Geometry check sheet. Reference: the model listing, model coordinates, mm. A direction names the side the tool comes from. Give positions to 0.01 mm unless a question says otherwise; leave off trailing zeros. Loops run counter-clockwise (first coordinate to the right, second up) from the corner with the lowest first, then second, coordinate; pieces in that order, holes last. Notation, with made-up numbers: (50.5, 23) -> (97.5, 23) arc R18 ccw to (97.5, 35) -> close; hole circle Ø5 at (71, 19). An arc over 180 degrees is marked (long way). One line per item, written item: value. Start each with the question number.
(1) Gauge pin test, flat ends, axial feed: pin 1 Ø2 at (x, z) = (164.35, 11.66) entering from +Y; pin 2 Ø4 at (y, z) = (2, -79) entering from +X; pin 3 Ø10.5 at (x, z) = (183, 0.5) entering from +Y; pin 4 Ø7.5 at (x, z) = (182.175, 0) entering from +Y. Record the tip position at first contact, or that the pin passes through.
(2) Scan lines: line 1 along Z through (x, y) = (23, 2.75) (3 decimals); line 2 along X through (y, z) = (0.5, -80) (3 decimals); line 3 along X through (y, z) = (7.25, 9.5). Record each from-to range of solid material in increasing order. Write a range as from..to.
(3) Sectioned sample at B-B, the plane z = -33.5. Record the cut outline in (x, y), then the cut area to 3 significant figures.
(4) Sectioned sample at A-A, the plane x = 1. Record the cut outline in (y, z) (3 decimals).
(5) Draft check along Z on faces 1 (the face through (146.106, 3.944, 46.261)), 2 (the face through (85, 0, 1)), 3 (the face through (188.4, 3.9, -22.3)), 4 (the face through (61.675, 4, -81)). Enter one of: pulls with the +Z half, pulls with the -Z half, needs draft (parallel to the pull), parting line crosses it, or undercut.
(6) Sectioned sample at C-C, the plane y = 2.75. State how many separate pieces and enclosed holes the cut face has, then the cut area to 3 significant figures.
(7) Sectioned sample at D-D, the plane z = 20. Record the cut outline in (x, y).
(8) Tool access check on faces 5 (the face through (114.091, 3.944, -88.146)), 6 (the face through (177.894, 7.014, 2.226)), 7 (the face through (-9.225, 4, 81)). Record the directions out of +Z, -Z, +X, -X, +Y, -Y that give a thin tool (end or side, any length) a straight path to the whole face; none if there is none.
from build123d import *

# Parameters (mm, degrees)
SALIENTE_EXTRUIR1_DEPTH = 8
CROQUIS2_R              = 1.825
CORTAR_EXTRUIR1_DEPTH   = 220.463870727
CROQUIS3_R              = 1.825
CORTAR_EXTRUIR2_DEPTH   = 220.463870727
CROQUIS4_W              = 103.75
CROQUIS4_H              = 91.75
CORTAR_EXTRUIR3_DEPTH   = 6.5
REDONDEO1_R             = 2.3
CROQUIS5_R              = 1.825
CORTAR_EXTRUIR4_DEPTH   = 220.463870727
CROQUIS20_W             = 70.9
CROQUIS20_H             = 14
CROQUIS20_W_2           = 13.452738683
CORTAR_EXTRUIR15_DEPTH  = 220.463870727
CROQUIS6_W              = 95.75
CROQUIS6_H              = 83.75
CORTAR_EXTRUIR5_DEPTH   = 220.414312556
CROQUIS9_R              = 1.825
CORTAR_EXTRUIR7_DEPTH   = 220.463870727
CROQUIS12_W             = 65
CROQUIS12_H             = 180
CORTAR_EXTRUIR9_DEPTH   = 220.463870727
REDONDEO2_R             = 8
CROQUIS14_R             = 1.825
CORTAR_EXTRUIR11_DEPTH  = 220.463870727
CROQUIS15_R             = 4.825
CORTAR_EXTRUIR12_DEPTH  = 2
CROQUIS16_W             = 11
CROQUIS16_H             = 47.47584408
CORTAR_EXTRUIR13_DEPTH  = 220.463870727
REDONDEO3_R             = 8
CROQUIS18_R             = 2.8
CORTAR_EXTRUIR14_DEPTH  = 4
CROQUIS21_W             = 108.962587205
CROQUIS21_H             = 10
SALIENTE_EXTRUIR9_DEPTH = 8
REDONDEO5_R             = 8
REDONDEO6_R             = 8
CROQUIS22_R             = 1.825
CORTAR_EXTRUIR16_DEPTH  = 215.858092703


with BuildPart() as part:
    # Croquis1 → Saliente-Extruir1 (new body)
    with BuildSketch(Plane(origin=(0, 0, 0), x_dir=(1, 0, 0), z_dir=(0, 1, 0))):
        with BuildLine():
            Line((0, 0), (200, 0))
            Line((200, 0), (200, 15.2))
            ThreePointArc((200, 15.2), (197.701163079, 20.938172036), (191.9990235, 23.3249845))
            ThreePointArc((191.9990235, 23.3249845), (148.666739026, 44.032184001), (120.7781513, 83.1307986))
            ThreePointArc((120.7781513, 83.1307986), (113.982057966, 88.196272982), (105.7, 90))
            Line((105.7, 90), (0, 90))
            Line((0, 90), (-79, 90))
            ThreePointArc((-79, 90), (-84.638146896, 87.675499941), (-86.999825594, 82.052824894))
            Line((-86.999825594, 82.052824894), (-86.999825594, 41.494023494))
            Line((-86.999825594, 41.494023494), (-86.999825594, 0))
            Line((-86.999825594, 0), (0, 0))
        make_face()
    extrude(amount=SALIENTE_EXTRUIR1_DEPTH)

    # Simetría2: part across plane


with BuildPart() as part_1:
    add(part.part)
    add(part.part.mirror(Plane(origin=(0, 8, 0), x_dir=(1, 0, 0), z_dir=(0, 0, -1))))

    # Croquis2 → Cortar-Extruir1 (cut, through all)
    with BuildSketch(Plane(origin=(0, 8, 0), x_dir=(1, 0, 0), z_dir=(0, 1, 0))):
        with Locations(Location((68.5, 81.35, 0), (0, 0, 270))):
            Circle(CROQUIS2_R)
        with Locations(Location((-16.05, 81.35, 0), (0, 0, 270))):
            Circle(CROQUIS2_R)
        with Locations(Location((68.5, -81.35, 0), (0, 0, 90))):
            Circle(CROQUIS2_R)
        with Locations(Location((-16.05, -81.35, 0), (0, 0, 90))):
            Circle(CROQUIS2_R)
    extrude(amount=-CORTAR_EXTRUIR1_DEPTH, mode=Mode.SUBTRACT)

    # Croquis3 → Cortar-Extruir2 (cut, through all)
    with BuildSketch(Plane(origin=(0, 8, 0), x_dir=(1, 0, 0), z_dir=(0, 1, 0))):
        with Locations(Location((-76.999825594, -46.75, 0), (0, 0, 270))):
            Circle(CROQUIS3_R)
        with Locations(Location((-34.999825594, -46.75, 0), (0, 0, 270))):
            Circle(CROQUIS3_R)
        with Locations(Location((-34.999825594, 46.75, 0), (0, 0, 90))):
            Circle(CROQUIS3_R)
        with Locations(Location((-76.999825594, 46.75, 0), (0, 0, 90))):
            Circle(CROQUIS3_R)
    extrude(amount=-CORTAR_EXTRUIR2_DEPTH, mode=Mode.SUBTRACT)

    # Croquis4 → Cortar-Extruir3 (cut)
    with BuildSketch(Plane(origin=(0, 8, 0), x_dir=(1, 0, 0), z_dir=(0, 1, 0))):
        with Locations((36.90017441, 0)):
            Rectangle(CROQUIS4_W, CROQUIS4_H)
    extrude(amount=-CORTAR_EXTRUIR3_DEPTH, mode=Mode.SUBTRACT)

    # Redondeo1
    redondeo1_edges = [part_1.edges().sort_by_distance(p)[0] for p in [
        (88.77517441, 4.75, -45.875),
        (88.77517441, 4.75, 45.875),
        (-14.97482559, 4.75, 45.875),
        (-14.97482559, 4.75, -45.875),
    ]]
    fillet(redondeo1_edges, radius=REDONDEO1_R)

    # Croquis5 → Cortar-Extruir4 (cut, through all)
    with BuildSketch(Plane(origin=(0, 8, 0), x_dir=(1, 0, 0), z_dir=(0, 1, 0))):
        with Locations(Location((98.35, 28.84, 0), (0, 0, 270))):
            Circle(CROQUIS5_R)
        with Locations(Location((98.35, -28.84, 0), (0, 0, 90))):
            Circle(CROQUIS5_R)
        with Locations(Location((164.35, 11.66, 0), (0, 0, 270))):
            Circle(CROQUIS5_R)
        with Locations(Location((164.35, -11.66, 0), (0, 0, 90))):
            Circle(CROQUIS5_R)
    extrude(amount=-CORTAR_EXTRUIR4_DEPTH, mode=Mode.SUBTRACT)

    # Croquis20 → Cortar-Extruir15 (cut, through all)
    with BuildSketch(Plane(origin=(0, 8, 0), x_dir=(1, 0, 0), z_dir=(0, 1, 0))):
        with Locations((26.225, -81)):
            Rectangle(CROQUIS20_W, CROQUIS20_H)
        with Locations((82.048805069, -81)):
            Rectangle(CROQUIS20_W_2, CROQUIS20_H)
        with Locations((82.048805069, 81)):
            Rectangle(CROQUIS20_W_2, CROQUIS20_H)
        with Locations((26.225, 81)):
            Rectangle(CROQUIS20_W, CROQUIS20_H)
    extrude(amount=-CORTAR_EXTRUIR15_DEPTH, mode=Mode.SUBTRACT)

    # Croquis6 → Cortar-Extruir5 (cut, through all)
    with BuildSketch(Plane(origin=(0, 1.5, 0), x_dir=(1, 0, 0), z_dir=(0, 1, 0))):
        with Locations((36.90017441, 0)):
            Rectangle(CROQUIS6_W, CROQUIS6_H)
    extrude(amount=-CORTAR_EXTRUIR5_DEPTH, mode=Mode.SUBTRACT)

    # Croquis9 → Cortar-Extruir7 (cut, through all)
    with BuildSketch(Plane(origin=(0, 8, 0), x_dir=(1, 0, 0), z_dir=(0, 1, 0))):
        with Locations(Location((-80.675393895, -75.767215538, 0), (0, 0, 270))):
            Circle(CROQUIS9_R)
        with Locations(Location((-58.52366486, -80.370640978, 0), (0, 0, 270))):
            Circle(CROQUIS9_R)
        with Locations(Location((-58.52366486, 80.370640978, 0), (0, 0, 90))):
            Circle(CROQUIS9_R)
        with Locations(Location((-80.675393895, 75.767215538, 0), (0, 0, 90))):
            Circle(CROQUIS9_R)
    extrude(amount=-CORTAR_EXTRUIR7_DEPTH, mode=Mode.SUBTRACT)

    # Croquis12 → Cortar-Extruir9 (cut, through all)
    with BuildSketch(Plane(origin=(0, 8, 0), x_dir=(1, 0, 0), z_dir=(0, 1, 0))):
        with Locations((-54.499825594, 0)):
            Rectangle(CROQUIS12_W, CROQUIS12_H)
    extrude(amount=-CORTAR_EXTRUIR9_DEPTH, mode=Mode.SUBTRACT)

    # Redondeo2
    redondeo2_edges = [part_1.edges().sort_by_distance(p)[0] for p in [
        (-21.999825594, 4, 90),
        (-21.999825594, 4, -90),
    ]]
    fillet(redondeo2_edges, radius=REDONDEO2_R)

    # Croquis14 → Cortar-Extruir11 (cut, through all)
    with BuildSketch(Plane(origin=(0, 8, 0), x_dir=(1, 0, 0), z_dir=(0, 1, 0))):
        with Locations(Location((182.175, 0, 0), (0, 0, 270))):
            Circle(CROQUIS14_R)
    extrude(amount=-CORTAR_EXTRUIR11_DEPTH, mode=Mode.SUBTRACT)

    # Croquis15 → Cortar-Extruir12 (cut)
    with BuildSketch(Plane(origin=(0, 8, 0), x_dir=(1, 0, 0), z_dir=(0, 1, 0))):
        with Locations(Location((182.175, 0, 0), (0, 0, 270))):
            Circle(CROQUIS15_R)
    extrude(amount=-CORTAR_EXTRUIR12_DEPTH, mode=Mode.SUBTRACT)

    # Croquis16 → Cortar-Extruir13 (cut, through all)
    with BuildSketch(Plane(origin=(0, 8, 0), x_dir=(1, 0, 0), z_dir=(0, 1, 0))):
        with Locations((195.5, 0)):
            Rectangle(CROQUIS16_W, CROQUIS16_H)
    extrude(amount=-CORTAR_EXTRUIR13_DEPTH, mode=Mode.SUBTRACT)

    # Redondeo3
    redondeo3_edges = [part_1.edges().sort_by_distance(p)[0] for p in [
        (190, 4, 23.73792204),
        (190, 4, -23.73792204),
    ]]
    fillet(redondeo3_edges, radius=REDONDEO3_R)

    # Croquis18 → Cortar-Extruir14 (cut)
    with BuildSketch(Plane.XZ):
        with Locations(Location((182.175, 0, 0), (0, 0, 270))):
            Circle(CROQUIS18_R)
    extrude(amount=-CORTAR_EXTRUIR14_DEPTH, mode=Mode.SUBTRACT)

    # Croquis21 → Saliente-Extruir9 (add)
    with BuildSketch(Plane(origin=(0, 8, 0), x_dir=(1, 0, 0), z_dir=(0, 1, 0))):
        with Locations((42.756293603, 95)):
            Rectangle(CROQUIS21_W, CROQUIS21_H)
        with Locations((42.756293603, -95)):
            Rectangle(CROQUIS21_W, CROQUIS21_H)
    extrude(amount=-SALIENTE_EXTRUIR9_DEPTH)

    # Redondeo5
    redondeo5_edges = [part_1.edges().sort_by_distance(p)[0] for p in [
        (-11.725, 4, -100),
        (97.237587205, 4, -100),
        (-11.725, 4, 100),
        (97.237587205, 4, 100),
    ]]
    fillet(redondeo5_edges, radius=REDONDEO5_R)

    # Redondeo6
    # the kernel refuses this fillet: 8 mm, written as the material it adds along each edge
    with BuildSketch(Plane(origin=(-11.725, 8, -90), x_dir=(0.09534974833302788, 0, -0.9954438334194594), z_dir=(0, -1, 0))) as redondeo6_piece_1:
        with BuildLine():
            CenterArc((6.539334701, -7.772851171), REDONDEO6_R, 103.686136853, 53.238021041)
            Line((-0.820560007, -4.637257147), (-1.556549478, -4.323697744))
            ThreePointArc((-1.556549478, -4.323697744), (-1.013259115, -2.188181311), (-0.796355067, 0.076279799))
            Line((-0.796355067, 0.076279799), (0.076279799, 0.796355067))
            ThreePointArc((0.076279799, 0.796355067), (2.067167466, 0.60565557), (4.457227725, 0.777285117))
            Line((4.457227725, 0.777285117), (4.646510177, 0))
        make_face()
    extrude(amount=8)
    with BuildSketch(Plane(origin=(97.237587205, 8, -90), x_dir=(-0.11597245427471743, 0, -0.9932524300748017), z_dir=(0, -1, 0))) as redondeo6_piece_2:
        with BuildLine():
            CenterArc((7.153649595, 7.714074532), REDONDEO6_R, 186.659717889, 67.975687163)
            Line((-0.792369846, 6.786294898), (-1.58697179, 6.693516934))
            Line((-1.58697179, 6.693516934), (-0.794601944, -0.092777963))
            Line((-0.794601944, -0.092777963), (0.092777963, -0.794601944))
            ThreePointArc((0.092777963, -0.794601944), (2.079282824, -0.562657036), (4.82199879, -0.771407453))
            Line((4.82199879, -0.771407453), (5.033967045, 0))
        make_face()
    extrude(amount=8)
    with BuildSketch(Plane(origin=(-11.725, 8, 90), x_dir=(-0.996830274314205, 0, -0.07955755281974515), z_dir=(0, -1, 0))) as redondeo6_piece_3:
        with BuildLine():
            CenterArc((6.514517354, -7.793662637), REDONDEO6_R, 103.04125749, 53.238021041)
            Line((-0.809619973, -4.575431382), (-1.542033706, -4.253608256))
            ThreePointArc((-1.542033706, -4.253608256), (-0.956579325, -1.930014506), (-0.797464219, 0.063646042))
            Line((-0.797464219, 0.063646042), (0.063646042, 0.797464219))
            ThreePointArc((0.063646042, 0.797464219), (2.331261063, 0.616484662), (4.528774303, 0.779366264))
            Line((4.528774303, 0.779366264), (4.709296399, 0))
        make_face()
    extrude(amount=8)
    with BuildSketch(Plane(origin=(97.237587205, 8, 90), x_dir=(1, 0, 0), z_dir=(0, -1, 0))) as redondeo6_piece_4:
        with BuildLine():
            CenterArc((6.832396974, 8), REDONDEO6_R, 202.024312837, 67.975687163)
            Line((-0.583801513, 5), (-1.325421362, 4.7))
            ThreePointArc((-1.325421362, 4.7), (-0.8, 2), (-0.8, 0))
            Line((-0.8, 0), (0, -0.8))
            Line((0, -0.8), (6.832396974, -0.8))
            Line((6.832396974, -0.8), (6.832396974, 0))
        make_face()
    extrude(amount=8)
    # the kernel refuses this fillet: 8 mm, written as the material it takes off along each edge

    # Croquis22 → Cortar-Extruir16 (cut, through all)
    with BuildSketch(Plane(origin=(0, 8, 0), x_dir=(1, 0, 0), z_dir=(0, 1, 0))):
        with Locations(Location((13.703094373, 94.859502658, 0), (0, 0, 270))):
            Circle(CROQUIS22_R)
        with Locations(Location((73.947520586, 94.859502658, 0), (0, 0, 90))):
            Circle(CROQUIS22_R)
        with Locations(Location((73.947520586, -94.859502658, 0), (0, 0, 270))):
            Circle(CROQUIS22_R)
        with Locations(Location((13.703094373, -94.859502658, 0), (0, 0, 90))):
            Circle(CROQUIS22_R)
    extrude(amount=-CORTAR_EXTRUIR16_DEPTH, mode=Mode.SUBTRACT)


solid = part_1.part
Calculated:
1. pin 1: passes through
1. pin 2: stops at x = 123.38
1. pin 3: stops at y = 8
1. pin 4: stops at y = 6
2. line 1: z = -100..-88, -74..-45.875, 45.875..74, 88..100
2. line 2: x = -22..-17.278, -14.822..-9.225, 61.675..67.272, 69.728..75.322, 88.775..122.045
2. line 3: x = -22..-14.97, 88.78..190
3. outline: (-22, 0) -> (-10.97, 0) -> (-10.97, 1.5) -> (-14.97, 1.5) -> (-14.97, 8) -> (-22, 8) -> close; (84.78, 0) -> (164.01, 0) -> (164.01, 8) -> (88.78, 8) -> (88.78, 1.5) -> (84.78, 1.5) -> close
3. area: 670 mm2
4. outline: (0, -100) -> (8, -100) -> (8, -88) -> (0, -88) -> close; (0, -74) -> (8, -74) -> (8, -45.875) -> (1.5, -45.875) -> (1.5, -41.875) -> (0, -41.875) -> close; (0, 41.875) -> (1.5, 41.875) -> (1.5, 45.875) -> (8, 45.875) -> (8, 74) -> (0, 74) -> close; (0, 88) -> (8, 88) -> (8, 100) -> (0, 100) -> close
5. face 1: pulls with the +Z half
5. face 2: needs draft
5. face 3: pulls with the -Z half
5. face 4: undercut
6. separate pieces: 1
6. enclosed holes: 18
6. area: 21,700 mm2
7. outline: (-22, 0) -> (-10.97, 0) -> (-10.97, 1.5) -> (-14.97, 1.5) -> (-14.97, 8) -> (-22, 8) -> close; (84.78, 0) -> (189.6, 0) -> (189.6, 8) -> (88.78, 8) -> (88.78, 1.5) -> (84.78, 1.5) -> close
8. face 5: -Z, +X, +Y, -Y
8. face 6: +Y
8. face 7: +Y, -Y
